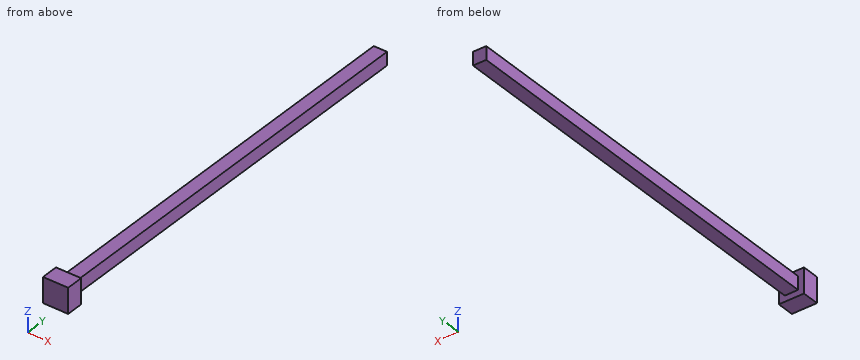
Autodesk Inventor part; units mm, degrees
ref_plane "YZ Plane" through (0, 0, 0) normal (1, 0, 0) x (0, 1, 0)
ref_plane "XZ Plane" through (0, 0, 0) normal (0, 1, 0) x (-1, 0, 0)
ref_plane "XY Plane" through (0, 0, 0) normal (0, 0, 1) x (1, 0, 0)
sketch "Szkic1" plane through (0, 0, 0) normal (0, 1, 0) x (-1, 0, 0)
  line L0 (-7.4, 7.4) -> (7.4, 7.4)
  line L1 (7.4, 7.4) -> (7.4, -7.4)
  line L2 (7.4, -7.4) -> (-7.4, -7.4)
  line L3 (-7.4, -7.4) -> (-7.4, 7.4)
  line L4 (-7.4, 7.4) -> (7.4, -7.4) construction
  line L5 (7.4, 7.4) -> (-7.4, -7.4) construction
  line L6 (3.9, 3.9) -> (-3.9, 3.9)
  line L7 (-3.9, 3.9) -> (-3.9, -3.9)
  line L8 (-3.9, -3.9) -> (3.9, -3.9)
  line L9 (3.9, -3.9) -> (3.9, 3.9)
  line L10 (3.9, 3.9) -> (-3.9, -3.9) construction
  line L11 (-3.9, 3.9) -> (3.9, -3.9) construction
  point P0 (0, 0)
  dimension "d0" = 14.8
  dimension "d1" = 14.8
  dimension "d7" = 7.8
  dimension "d8" = 7.8
extrude "Wyciągnięcie proste1" add sketch "Szkic1" against normal blind 10 contours L0 L1 L2 L3 | L9 L8 L7 L6
extrude "Wyciągnięcie proste2" add sketch "Szkic1" along normal blind 240 contours L9 L8 L7 L6
properties part number "podstawa_rod"
Can you work these out from the model? Positions are in its coordinate system, mm. Coordinates: 2 decimals unless noted, no trailing zeros. Order: outer loops, then holes, each group sorted by start corner. A loop starts at its lowest first (then second) coordinate and runs counter-clockwise, first axis right, second up. Notation, with made-up numbers: (-14, -25) - (17, -25) arc R15 cw to (17, -2) - close; hole circle Ø5 at (55, 9.25). An arc over 180 degrees is marked (long way). Answer in a Markdown table with one row per item.
1. Suppose I cut it at A-A (x = 1.25). Please give me the cut outline in (y, z).
Reply:
| item | result |
|---|---|
| outline | (-10, -7.4) - (0, -7.4) - (0, -3.9) - (240, -3.9) - (240, 3.9) - (0, 3.9) - (0, 7.4) - (-10, 7.4) - close |
2. For pin 1 (4 mm diameter, centred on y = 111.5, z = 1.5, fed in from -X); pin 2 (6 mm diameter, centred on x = -0.5, y = 62, fed in from +Z); pin 3 (1 mm diameter, centred on x = 3, z = -5.5, fed in from +Y), each with a flat end and sliding along its axis, tell me the tip position at first contact or that it passes through.
Reply:
| item | result |
|---|---|
| pin 1 | stops at x = -3.9 |
| pin 2 | stops at z = 3.9 |
| pin 3 | stops at y = 0 |
3. Suppose I cut it at B-B (z = 1.5). Please give me the cut outline in (x, y).
Reply:
| item | result |
|---|---|
| outline | (-7.4, -10) - (7.4, -10) - (7.4, 0) - (3.9, 0) - (3.9, 240) - (-3.9, 240) - (-3.9, 0) - (-7.4, 0) - close |
4. Suppose I cut it at C-C (y = 45). Please give me the cut outline in (x, z).
Reply:
| item | result |
|---|---|
| outline | (-3.9, -3.9) - (3.9, -3.9) - (3.9, 3.9) - (-3.9, 3.9) - close |
5. If I drill on line 1 along Z through (x, y) = (-2.25, 224); line 2 along Y through (x, z) = (2.5, -5.5), over which ranges is the centre line in solid material (lowest first)?
Reply:
| item | result |
|---|---|
| line 1 | z = -3.9 to 3.9 |
| line 2 | y = -10 to 0 |
